Build history of the part. All positions in model axes, mm. A direction names the side the tool comes from. Round coordinates to 2 decimals unless told otherwise and drop trailing zeros. Order: outer loops, then holes, each group sorted by start corner. A loop starts at its lowest first (then second) coordinate and runs counter-clockwise, first axis right, second up. Notation, with made-up numbers: (19, 28.25) -> (64, 28.25) arc R15 ccw to (64, 38.25) -> close; hole circle Ø7 at (15.5, 3.25). An arc over 180 degrees is marked (long way). Answer as a JSON object with one key per item and string values.
from build123d import *

# Parameters (mm, degrees)
BOSS_EXTRUDE1_OUTLINE_R    = 2.55
BOSS_EXTRUDE1_OUTLINE_R_2  = 2.621431339
BOSS_EXTRUDE1_OUTLINE_R_3  = 2.017902989
BOSS_EXTRUDE1_OUTLINE_R_4  = 2.1
BOSS_EXTRUDE1_OUTLINE_R_5  = 2.538142432
BOSS_EXTRUDE1_OUTLINE_R_6  = 2.478866387
BOSS_EXTRUDE1_OUTLINE_R_7  = 2.709196321
BOSS_EXTRUDE1_OUTLINE_R_8  = 2.625839509
BOSS_EXTRUDE1_OUTLINE_R_9  = 3.6
BOSS_EXTRUDE1_OUTLINE_R_10 = 2.614760952
BOSS_EXTRUDE1_DEPTH        = 6
SKETCH2_R                  = 6
SKETCH2_R_2                = 4.5
CUT_EXTRUDE1_DEPTH         = 1.5


# Read off the part's stored shape, not the designer's step: Boss-Extrude1
with BuildPart() as part:
    # Boss-Extrude1 outline → Boss-Extrude1 (new body)
    with BuildSketch(Plane.XY):
        with BuildLine():
            Line((-2.55, 0), (-2.55, 4.870526086))
            ThreePointArc((-2.55, 4.870526086), (0, 7.420526086), (2.55, 4.870526086))
            Line((2.55, 4.870526086), (2.55, 0))
            Line((2.55, 0), (38.76, 0))
            Line((38.76, 0), (38.76, 72.51))
            ThreePointArc((38.76, 72.51), (37.295533906, 76.045533906), (33.76, 77.51))
            Line((33.76, 77.51), (-33.76, 77.51))
            ThreePointArc((-33.76, 77.51), (-37.295533906, 76.045533906), (-38.76, 72.51))
            Line((-38.76, 72.51), (-38.76, 0))
            Line((-38.76, 0), (-2.55, 0))
        make_face()
        with Locations((-30.09, 8.75)):
            Circle(BOSS_EXTRUDE1_OUTLINE_R, mode=Mode.SUBTRACT)
        with Locations((-10.01, 5.02)):
            Circle(BOSS_EXTRUDE1_OUTLINE_R_2, mode=Mode.SUBTRACT)
        with Locations((-10.01, 15.02)):
            Circle(BOSS_EXTRUDE1_OUTLINE_R_3, mode=Mode.SUBTRACT)
        with Locations((-30.09, 28.75)):
            Circle(BOSS_EXTRUDE1_OUTLINE_R_4, mode=Mode.SUBTRACT)
        with Locations((-20, 20)):
            Circle(BOSS_EXTRUDE1_OUTLINE_R_4, mode=Mode.SUBTRACT)
        with Locations((-20, 38.75)):
            Circle(BOSS_EXTRUDE1_OUTLINE_R_5, mode=Mode.SUBTRACT)
        with Locations((-8.75, 28.75)):
            Circle(BOSS_EXTRUDE1_OUTLINE_R_6, mode=Mode.SUBTRACT)
        with Locations((10.01, 5.02)):
            Circle(BOSS_EXTRUDE1_OUTLINE_R_2, mode=Mode.SUBTRACT)
        with Locations((0, 15.02)):
            Circle(BOSS_EXTRUDE1_OUTLINE_R_7, mode=Mode.SUBTRACT)
        with Locations((10.01, 15.02)):
            Circle(BOSS_EXTRUDE1_OUTLINE_R_3, mode=Mode.SUBTRACT)
        with Locations((30.09, 8.75)):
            Circle(BOSS_EXTRUDE1_OUTLINE_R, mode=Mode.SUBTRACT)
        with Locations((8.75, 28.75)):
            Circle(BOSS_EXTRUDE1_OUTLINE_R_6, mode=Mode.SUBTRACT)
        with Locations((20, 20)):
            Circle(BOSS_EXTRUDE1_OUTLINE_R_4, mode=Mode.SUBTRACT)
        with Locations((30.09, 28.75)):
            Circle(BOSS_EXTRUDE1_OUTLINE_R_4, mode=Mode.SUBTRACT)
        with Locations((20, 38.75)):
            Circle(BOSS_EXTRUDE1_OUTLINE_R_5, mode=Mode.SUBTRACT)
        with Locations((-30.09, 48.75)):
            Circle(BOSS_EXTRUDE1_OUTLINE_R_4, mode=Mode.SUBTRACT)
        with Locations((-14.25, 48.75)):
            Circle(BOSS_EXTRUDE1_OUTLINE_R, mode=Mode.SUBTRACT)
        with Locations((-20, 58.76)):
            Circle(BOSS_EXTRUDE1_OUTLINE_R_4, mode=Mode.SUBTRACT)
        with Locations((-30.09, 68.75)):
            Circle(BOSS_EXTRUDE1_OUTLINE_R_4, mode=Mode.SUBTRACT)
        with Locations((-14.25, 68.75)):
            Circle(BOSS_EXTRUDE1_OUTLINE_R, mode=Mode.SUBTRACT)
        with Locations((0, 48.75)):
            Circle(BOSS_EXTRUDE1_OUTLINE_R_8, mode=Mode.SUBTRACT)
        with Locations((14.25, 48.75)):
            Circle(BOSS_EXTRUDE1_OUTLINE_R_9, mode=Mode.SUBTRACT)
        with Locations((30.09, 48.75)):
            Circle(BOSS_EXTRUDE1_OUTLINE_R_4, mode=Mode.SUBTRACT)
        with Locations((0, 68.75)):
            Circle(BOSS_EXTRUDE1_OUTLINE_R_10, mode=Mode.SUBTRACT)
        with Locations((14.25, 68.75)):
            Circle(BOSS_EXTRUDE1_OUTLINE_R_9, mode=Mode.SUBTRACT)
        with Locations((20, 58.76)):
            Circle(BOSS_EXTRUDE1_OUTLINE_R_4, mode=Mode.SUBTRACT)
        with Locations((30.09, 68.75)):
            Circle(BOSS_EXTRUDE1_OUTLINE_R_4, mode=Mode.SUBTRACT)
    extrude(amount=BOSS_EXTRUDE1_DEPTH)

    # Sketch2 → Cut-Extrude1 (cut)
    with BuildSketch(Plane.XY.offset(6)):
        with Locations((14.25, 68.75)):
            Circle(SKETCH2_R)
        with Locations((14.25, 48.75)):
            Circle(SKETCH2_R)
        with Locations((-14.25, 48.75)):
            Circle(SKETCH2_R_2)
        with Locations((-14.25, 68.75)):
            Circle(SKETCH2_R_2)
        with BuildLine():
            Line((9.95, -20), (-9.95, -20))
            ThreePointArc((-9.95, -20), (-13.485533906, -18.535533906), (-14.95, -15))
            Line((-14.95, -15), (-14.95, 15))
            ThreePointArc((-14.95, 15), (-13.485533906, 18.535533906), (-9.95, 20))
            Line((-9.95, 20), (9.95, 20))
            ThreePointArc((9.95, 20), (13.485533906, 18.535533906), (14.95, 15))
            Line((14.95, 15), (14.95, -15))
            ThreePointArc((14.95, -15), (13.485533906, -18.535533906), (9.95, -20))
        make_face()
    extrude(amount=-CUT_EXTRUDE1_DEPTH, mode=Mode.SUBTRACT)

    # Mirror1: part across plane


with BuildPart() as part_1:
    add(part.part)
    add(part.part.mirror(Plane(origin=(0, 0, 6), x_dir=(0, 0, 1), z_dir=(0, 1, 0))))


solid = part_1.part
1) Flat gauge pins, fed straight in: pin 1 Ø2.5 at (x, y) = (-20, 58.76) entering from -Z; pin 2 Ø11 at (x, y) = (14.25, -48.75) entering from +Z. Where does each tip first touch, or does it go through?
Checked values:
{"pin 1": "passes through", "pin 2": "stops at z = 4.5"}
2) Cut at A-A, the plane y = 58.76. Give the cut face in (x, z).
Checked values:
{"outline": "(-38.76, 0) -> (-22.1, 0) -> (-22.1, 6) -> (-38.76, 6) -> close; (-17.9, 0) -> (17.9, 0) -> (17.9, 6) -> (-17.9, 6) -> close; (22.1, 0) -> (38.76, 0) -> (38.76, 6) -> (22.1, 6) -> close"}
3) Which spindle directions (+Z, -Z, +X, -X, +Y, -Y) get a long thin tool onto all of the face, cutting with end or side? Do faces 4 (the face through (-7.61, 26.55, 2.96)), 5 (the face through (-14.84, -73.21, 5.26)). Say none if no direction does.
Checked values:
{"face 4": "+Z, -Z", "face 5": "+Z"}
4) Cut at C-C, the plane y = 28.75. Give the cut face in (x, z), plus the area to 3 significant figures.
Checked values:
{"outline": "(-38.76, 0) -> (-32.19, 0) -> (-32.19, 6) -> (-38.76, 6) -> close; (-27.99, 0) -> (-11.23, 0) -> (-11.23, 6) -> (-27.99, 6) -> close; (-6.27, 0) -> (6.27, 0) -> (6.27, 6) -> (-6.27, 6) -> close; (11.23, 0) -> (27.99, 0) -> (27.99, 6) -> (11.23, 6) -> close; (32.19, 0) -> (38.76, 0) -> (38.76, 6) -> (32.19, 6) -> close", "area": "355 mm²"}
5) Cut at B-B, the plane y = -68.75. Count the separate pieces of the cut face and the enclosed holes in it, plus the area to 3 significant figures.
Checked values:
{"separate pieces": "6", "enclosed holes": "0", "area": "296 mm²"}
6) Probe L1, parallel to X at y = -28.75, z = 1.95; L2, parallel to X at y = -15, z = 4.2; L3, parallel to X at y = -48.75, z = 1.75. List the from-to ranges inside material, lowest first. Write a range as from..to.
Checked values:
{"L1": "x = -38.76..-32.19, -27.99..-11.23, -6.27..6.27, 11.23..27.99, 32.19..38.76", "L2": "x = -38.76..-12.03, -7.99..-2.71, 2.71..7.99, 12.03..38.76", "L3": "x = -38.76..-32.19, -27.99..-16.8, -11.7..-2.63, 2.63..10.65, 17.85..27.99, 32.19..38.76"}
7) Pull direction Y, two halves, no side cores. Call faces 1 (the face through (-0.06, -7.42, 2.22)), 2 (the face through (11.22, 2.694, 2.218)), 3 (the face through (37.33, 76.01, 2.96)): pulls with the +Y half, pulls with the -Y half, needs draft (parallel to the pull), parting line crosses it, or undercut.
Checked values:
{"face 1": "undercut", "face 2": "undercut", "face 3": "pulls with the +Y half"}
